The model under review builds one solid part; all positions refer to its coordinate system, in mm. A direction names the side the tool comes from. Give positions to 0.01 mm unless a question says otherwise; leave off trailing zeros. Write each loop counter-clockwise with the first axis right and the second up, starting at its lowest first coordinate (ties: lowest second). Pieces come first, ordered by that corner, then holes. Notation, with made-up numbers: M 64.5,47 L 93.5,47 A20 ccw 93.5,69 Z; hole C 63.5,0 d7. An arc over 180 degrees is marked long. Write item = value, one per line. Start each with the question number.
```python
from build123d import *

# Parameters (mm, degrees)
SKETCH_R             = 18
PAD_DEPTH            = 36
SKETCH001_R          = 14
POCKET_DEPTH         = 36.001
SKETCH004_W          = 15.214258
SKETCH004_H          = 18
PAD001_DEPTH         = 1
SKETCH005_W          = 11.214258
SKETCH005_H          = 14
PAD002_DEPTH         = 2
POCKET001_DEPTH      = 33
POCKET002_DEPTH      = 18.001
POCKET002_DEPTH_BACK = -34.31454
SKETCH007_W          = 4
SKETCH007_H          = 2
PAD003_DEPTH         = 1
SKETCH008_W          = 11.214258
SKETCH008_H          = 12
PAD004_DEPTH         = 3


with BuildPart() as part:
    # Sketch → Pad (new body)
    with BuildSketch(Plane.XY):
        Circle(SKETCH_R)
    extrude(amount=PAD_DEPTH)

    # Sketch001 → Pocket (cut, through all)
    with BuildSketch(Plane.XY):
        Circle(SKETCH001_R)
    extrude(amount=POCKET_DEPTH, mode=Mode.SUBTRACT)

    # Sketch004 → Pad001 (join)
    with BuildSketch(Plane.XY.offset(1)):
        with Locations((0, -25.31354)):
            Rectangle(SKETCH004_W, SKETCH004_H)
    extrude(amount=PAD001_DEPTH)

    # Sketch005 → Pad002 (join)
    with BuildSketch(Plane.XY):
        with Locations((0, -25.31354)):
            Rectangle(SKETCH005_W, SKETCH005_H)
    extrude(amount=PAD002_DEPTH)

    # Sketch002 → Pocket001 (cut, symmetric)
    with BuildSketch(Plane.XZ):
        with BuildLine():
            Line((-40, -10), (40, -10))
            Line((40, -10), (40, 18))
            Line((40, 18), (22, 18))
            ThreePointArc((22, 18), (19.18561, 16.995366), (17.643564, 14.435644))
            ThreePointArc((-17.643564, 14.435644), (0, 0), (17.643564, 14.435644))
            ThreePointArc((-17.643564, 14.435644), (-19.18561, 16.995366), (-22, 18))
            Line((-22, 18), (-40, 18))
            Line((-40, 18), (-40, -10))
        make_face()
    extrude(amount=POCKET001_DEPTH, both=True, mode=Mode.SUBTRACT)

    # Sketch003 → Pocket002 (cut, two sides)
    with BuildSketch(Plane.XZ) as pocket002_sk:
        with BuildLine():
            Line((-30, 36), (30, 36))
            Line((30, 36), (30, 18))
            Line((30, 18), (20.4369, 18))
            ThreePointArc((20.4369, 18), (17.514273, 17.079952), (15.645716, 14.651632))
            ThreePointArc((-15.645716, 14.651632), (0, 2), (15.645716, 14.651632))
            ThreePointArc((-15.645716, 14.651632), (-17.514273, 17.079952), (-20.4369, 18))
            Line((-20.4369, 18), (-30, 18))
            Line((-30, 18), (-30, 36))
        make_face()
    extrude(amount=-POCKET002_DEPTH, mode=Mode.SUBTRACT)
    extrude(pocket002_sk.sketch, amount=-POCKET002_DEPTH_BACK, mode=Mode.SUBTRACT)

    # Sketch007 → Pad003 (join, symmetric)
    with BuildSketch(Plane.XY):
        with Locations((0, 16)):
            Rectangle(SKETCH007_W, SKETCH007_H)
    extrude(amount=PAD003_DEPTH, both=True)

    # Sketch008 → Pad004 (join)
    with BuildSketch(Plane.XY.offset(2)):
        with Locations((0, -26.31354)):
            Rectangle(SKETCH008_W, SKETCH008_H)
    extrude(amount=-PAD004_DEPTH)


solid = part.part
```
Item 1: The part is to be moulded in two halves that separate along X. For faces 5 (the cylindrical face through (-0.1, -18, 0.6)), 6 (the cylindrical face through (-16.304, 0.125, 15.89)), 7 (the cylindrical face through (-17.75, -0.05, 14.85)), say which applies: released by +X, released by -X, zero draft, split by the parting line, or undercut.
Item 2: We need section C-C, the plane x = 7. Write out the cut boundary in (y, z).
Item 3: We need section A-A, the plane z = 5.5. Write out the cut boundary in (x, y), and give its area (3 significant figures).
Item 4: Clearance check with flat-ended pins moving along their axes: P1, Ø0.6, axis at y = 16, z = -0.5, coming from the +X side; P2, Ø1.2, axis at x = -0.5, z = -0.5, coming from the +Y side; P3, Ø4, axis at y = -16.5, z = 6.5, coming from the +X side; P4, Ø10, axis at x = -6, z = 12.5, coming from the +Y side. State where each tip first meets the part, or that it passes through.
Item 5: To check wall thickness, follow probe 1 along X at (y, z) = (-6, 7.75); probe 2 along Z at (x, y) = (2, -19); probe 3 along X at (y, z) = (0, 8). State the ranges of each line that lie inside material, in increasing order. Write a range as [from, to].
Item 6: For faces 1 (the flat face through (2, 16, -0.4)), 2 (the cylindrical face through (0, -19, 0)), 3 (the flat face through (-0.1, -18.314, 0.6)), 4 (the cylindrical face through (16.335, -0.125, 15.931)), list the 3-axis set-ups (+Z, -Z, +X, -X, +Y, -Y) from which the entire face can be reached by the end or side of a thin tool; tool diameter is ignored.
Item 7: We need section B-B, the plane y = -8. Write out the cut boundary in (x, z).
Item 8: We need section D-D, the plane y = -29.5. Write out the cut boundary in (x, z).
Worked out:
q1.face_5 = split by the parting line
q1.face_6 = undercut
q1.face_7 = released by -X
q2.outline = M -34.31,1 L -33,1 L -33,1.42 L -12.12,1.42 L -12.12,3.61 L -16.58,3.61 L -16.58,2 L -34.31,2 Z; M 12.12,1.42 L 16.58,1.42 L 16.58,3.61 L 12.12,3.61 Z
q3.outline = M -12.95,-12.5 A18 ccw -9.99,-14.97 L -9.99,-9.81 A14 cw -12.95,-5.32 Z; M -12.95,5.32 A14 cw -9.99,9.81 L -9.99,14.97 A18 ccw -12.95,12.5 Z; M 9.99,-14.97 A18 ccw 12.95,-12.5 L 12.95,-5.32 A14 cw 9.99,-9.81 Z; M 9.99,9.81 A14 cw 12.95,5.32 L 12.95,12.5 A18 ccw 9.99,14.97 Z
q3.area = 70.5 mm²
q4.P1 = 2
q4.P2 = 18
q4.P3 = 10.58
q4.P4 = through
q5.probe_1 = [-14.8, -12.65], [12.65, 14.8]
q5.probe_2 = [0.11, 2]
q5.probe_3 = [-14.97, -14], [14, 14.97]
q6.face_1 = -Z, +X, +Y
q6.face_2 = -Z
q6.face_3 = -Z, +X, -X
q6.face_4 = +Z, +Y, -Y
q7.outline = M -16.12,10 A18 ccw -11.49,4.14 L -11.49,6.86 A16 cw -15.65,14.65 A5.1 ccw -16.12,15.62 Z; M 11.49,4.14 A18 ccw 16.12,10 L 16.12,15.62 A5.1 ccw 15.65,14.65 A16 cw 11.49,6.86 Z
q8.outline = M -7.61,1.69 A18 ccw -5.92,1 L -5.61,1 L -5.61,-1 L 5.61,-1 L 5.61,1 L 5.92,1 A18 ccw 7.61,1.69 L 7.61,2 L -7.61,2 Z
